The listing builds one solid part. Answer for the finished solid, in the listing's coordinates (mm). Face numbers are marked on the shaded views. A direction names the side the tool comes from. Give positions to 0.01 mm unless a question says otherwise; leave off trailing zeros. Write each loop counter-clockwise with the first axis right and the second up, starting at its lowest first coordinate (ties: lowest second). Pieces come first, ordered by that corner, then holes. Notation, with made-up numbers: (29.25, 37.5) -> (72.25, 37.5) arc R26 ccw to (72.25, 57.5) -> close; hole circle Ø8 at (80, 22.5). An arc over 180 degrees is marked (long way). Put each result on its own line as item: value. Start each with the question number.
1) Flat-ended cylindrical pins translate along their axes: pin 1 Ø2.5 at (y, z) = (12, 22.5) entering from -X; pin 2 Ø5 at (x, z) = (5.5, -3) entering from +Y; pin 3 Ø2 at (x, y) = (22.5, 1) entering from +Z. Find the tip coordinate at first contact, or state that the pin passes through.
2) A cutting plane is placed at B-B (x = -10.5). Give the number of separate pieces and of enclosed holes in the cut face, then the cut area to 3 significant figures.
3) A cutting plane is placed at C-C (x = 24). Write down the section's boundary in (y, z).
4) Find the intervals of material crossed by line 1 along X through (y, z) = (0.75, 10.5); line 2 along Y through (x, z) = (24.5, -7.45); line 3 along Z through (x, y) = (-24, 0.95), in increasing order. Write a range as from..to.
5) For the marked faces 1, 2 and 3, determine the directions among +Z, -Z, +X, -X, +Y, -Y from which every point of the face is accessible in a straight line to the end or side of a thin tool.
6) A cutting plane is placed at A-A (y = 17). Write down the section's boundary in (x, z).
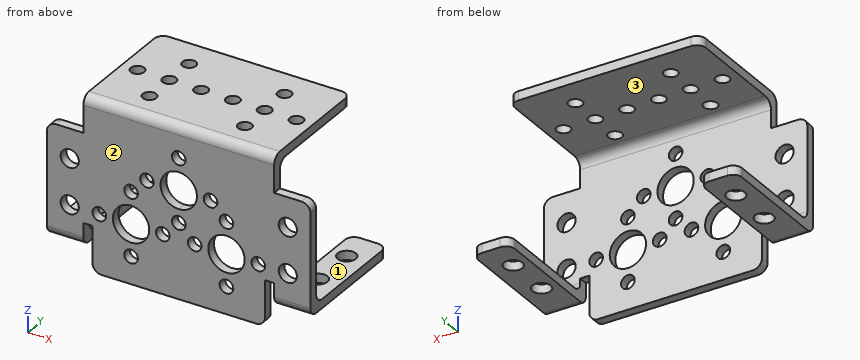
from build123d import *

# Parameters (mm, degrees)
SKETCH_1_R          = 1.5
SKETCH_1_R_2        = 2
SKETCH_1_R_3        = 4
EXTRUDE_1_DEPTH     = 2
SKETCH_2_W          = 8
SKETCH_2_H          = 2
EXTRUDE_2_DEPTH     = 25
SKETCH_3_R          = 2
CUT_EXTRUDE_1_DEPTH = 51.002499938
SKETCH_4_W          = 42
SKETCH_4_H          = 2
EXTRUDE_3_DEPTH     = 25
SKETCH_5_R          = 1.5
CUT_EXTRUDE_2_DEPTH = 25
FILLET_1_R          = 2
FILLET_2_R          = 2


with BuildPart() as part:
    # 草图1 → 凸台-拉伸1 (new body)
    with BuildSketch(Plane(origin=(0, 0, 0), x_dir=(1, 0, 0), z_dir=(0, 1, 0))):
        with BuildLine():
            Line((0, -19), (0, -24.5))
            Line((0, -24.5), (21, -24.5))
            Line((21, -24.5), (21, -16.5))
            Line((21, -16.5), (27, -16.5))
            ThreePointArc((27, -16.5), (28.414213562, -15.914213562), (29, -14.5))
            Line((29, -14.5), (29, 8))
            Line((29, 8), (21, 8))
            Line((21, 8), (21, 3))
            Line((21, 3), (19, 3))
            Line((19, 3), (19, 11))
            ThreePointArc((19, 11), (18.414213562, 12.414213562), (17, 13))
            Line((17, 13), (0, 13))
            Line((0, 13), (0, -2))
            ThreePointArc((0, -2), (1.060660172, -2.439339828), (1.5, -3.5))
            ThreePointArc((1.5, -3.5), (1.060660172, -4.560660172), (0, -5))
            Line((0, -5), (0, -6.5))
            ThreePointArc((0, -6.5), (2.828427125, -7.671572875), (4, -10.5))
            ThreePointArc((4, -10.5), (2.828427125, -13.328427125), (0, -14.5))
            Line((0, -14.5), (0, -16))
            ThreePointArc((0, -16), (1.060660172, -16.439339828), (1.5, -17.5))
            ThreePointArc((1.5, -17.5), (1.060660172, -18.560660172), (0, -19))
        make_face()
        with Locations(Location((7, -10.5, 0), (0, 0, 270))):
            Circle(SKETCH_1_R, mode=Mode.SUBTRACT)
        with Locations(Location((10.5, -7, 0), (0, 0, 270))):
            Circle(SKETCH_1_R, mode=Mode.SUBTRACT)
        with Locations(Location((24, -10, 0), (0, 0, 270))):
            Circle(SKETCH_1_R_2, mode=Mode.SUBTRACT)
        with Locations(Location((3.5, 0, 0), (0, 0, 270))):
            Circle(SKETCH_1_R, mode=Mode.SUBTRACT)
        with Locations(Location((10.5, 0, 0), (0, 0, 270))):
            Circle(SKETCH_1_R_3, mode=Mode.SUBTRACT)
        with Locations(Location((10.5, 7, 0), (0, 0, 270))):
            Circle(SKETCH_1_R, mode=Mode.SUBTRACT)
        with Locations(Location((17.5, 0, 0), (0, 0, 270))):
            Circle(SKETCH_1_R, mode=Mode.SUBTRACT)
        with Locations(Location((24, 0, 0), (0, 0, 270))):
            Circle(SKETCH_1_R_2, mode=Mode.SUBTRACT)
    extrude_1 = extrude(amount=EXTRUDE_1_DEPTH)

    # 草图2 → 凸台-拉伸2 (add)
    with BuildSketch(Plane(origin=(0, 2, 0), x_dir=(1, 0, 0), z_dir=(0, 1, 0))):
        with Locations((25, 7)):
            Rectangle(SKETCH_2_W, SKETCH_2_H)
    extrude_2 = extrude(amount=EXTRUDE_2_DEPTH)

    # 草图3 → 切除-拉伸1 (cut, through all)
    with BuildSketch(Plane.XY.offset(-6)):
        with Locations((24.5, 10)):
            Circle(SKETCH_3_R)
        with Locations((24.5, 20)):
            Circle(SKETCH_3_R)
        with BuildLine():
            ThreePointArc((21, 25), (21.585786438, 26.414213562), (23, 27))
            Line((23, 27), (21, 27))
            Line((21, 27), (21, 25))
        make_face()
        with BuildLine():
            Line((29, 27), (27, 27))
            ThreePointArc((27, 27), (28.414213562, 26.414213562), (29, 25))
            Line((29, 25), (29, 27))
        make_face()
    cut_extrude_1 = extrude(amount=-CUT_EXTRUDE_1_DEPTH, mode=Mode.SUBTRACT)

    # 镜向1: 凸台-拉伸1, 凸台-拉伸2, 切除-拉伸1 across plane
    add(extrude_1.mirror(Plane(origin=(0, 2, 0), x_dir=(0, 0, 1), z_dir=(1, 0, 0))))
    add(extrude_2.mirror(Plane(origin=(0, 2, 0), x_dir=(0, 0, 1), z_dir=(1, 0, 0))))
    add(cut_extrude_1.mirror(Plane(origin=(0, 2, 0), x_dir=(0, 0, 1), z_dir=(1, 0, 0))), mode=Mode.SUBTRACT)

    # 草图4 → 凸台-拉伸3 (add)
    with BuildSketch(Plane(origin=(0, 2, 0), x_dir=(1, 0, 0), z_dir=(0, 1, 0))):
        with Locations((0, -23.5)):
            Rectangle(SKETCH_4_W, SKETCH_4_H)
    extrude(amount=EXTRUDE_3_DEPTH)

    # 草图5 → 切除-拉伸2 (cut)
    with BuildSketch(Plane.XY.offset(24.5)):
        with Locations((-10.5, 13.5)):
            Circle(SKETCH_5_R)
        with Locations((10.5, 13.5)):
            Circle(SKETCH_5_R)
        with Locations((-10.5, 20.5)):
            Circle(SKETCH_5_R)
        with Locations((-3.5, 13.5)):
            Circle(SKETCH_5_R)
        with Locations((-10.5, 6.5)):
            Circle(SKETCH_5_R)
        with Locations((-17.5, 13.5)):
            Circle(SKETCH_5_R)
        with Locations((10.5, 20.5)):
            Circle(SKETCH_5_R)
        with Locations((17.5, 13.5)):
            Circle(SKETCH_5_R)
        with Locations((10.5, 6.5)):
            Circle(SKETCH_5_R)
        with Locations((3.5, 13.5)):
            Circle(SKETCH_5_R)
    extrude(amount=-CUT_EXTRUDE_2_DEPTH, mode=Mode.SUBTRACT)

    # 圆角1
    fillet_1_edges = [part.edges().sort_by_distance(p)[0] for p in [
        (-21, 27, 23.5),
        (21, 27, 23.5),
    ]]
    fillet(fillet_1_edges, radius=FILLET_1_R)

    # 圆角2
    fillet_2_edges = [part.edges().sort_by_distance(p)[0] for p in [
        (-25, 0, -8),
        (-25, 2, -6),
        (0, 2, 22.5),
        (25, 0, -8),
        (0, 0, 24.5),
        (25, 2, -6),
    ]]
    fillet(fillet_2_edges, radius=FILLET_2_R)


solid = part.part
Reply:
1. pin 1: stops at x = -21
1. pin 2: stops at y = 2
1. pin 3: stops at z = 16.5
2. separate pieces: 7
2. enclosed holes: 0
2. area: 79.0 mm2
3. outline: (0, -6) arc R2 ccw to (2, -8) -> (8.06, -8) -> (8.06, -6) -> (4, -6) arc R2 cw to (2, -4) -> (2, -2) -> (0, -2) -> close; (0, 2) -> (2, 2) -> (2, 8) -> (0, 8) -> close; (0, 12) -> (2, 12) -> (2, 16.5) -> (0, 16.5) -> close; (11.94, -8) -> (18.06, -8) -> (18.06, -6) -> (11.94, -6) -> close; (21.94, -8) -> (27, -8) -> (27, -6) -> (21.94, -6) -> close
4. line 1: x = -29..-25.94, -22.06..-8.5, -5.5..-4, 4..5.5, 8.5..22.06, 25.94..29
4. line 2: y = 0.62..8, 12..18, 22..27
4. line 3: z = -7.7..-2, 2..8, 12..16.5
5. face 1: +Z, +X, -X, +Y
5. face 2: +Z, -Z, +X, -X, -Y
5. face 3: -Z, +X, -X, +Y
6. outline: (-29, -8) -> (-21, -8) -> (-21, -6) -> (-29, -6) -> close; (-21, 22.5) -> (21, 22.5) -> (21, 24.5) -> (-21, 24.5) -> close; (21, -8) -> (29, -8) -> (29, -6) -> (21, -6) -> close
